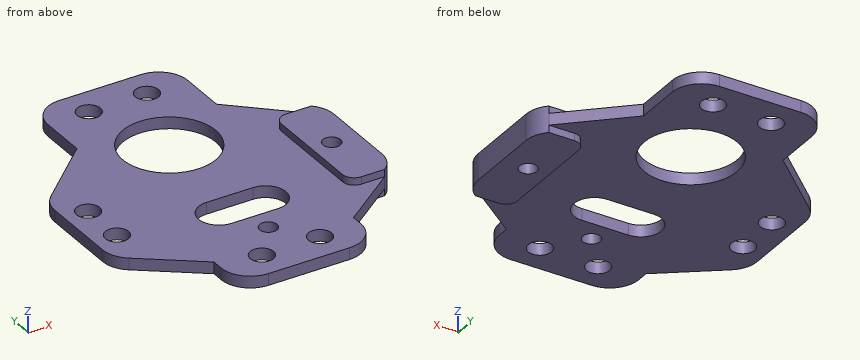
from build123d import *

# Parameters (mm, degrees)
SKETCH_1_R               = 2
SKETCH_1_R_2             = 8
SKETCH_1_R_3             = 1.5
EXTRUDE_1_DEPTH          = 2
EXTRUDE_2_DEPTH          = 3.25
CUT_EXTRUDE_1_DEPTH      = 39.603141342
CUT_EXTRUDE_1_DEPTH_BACK = 39.603141342
SKETCH_3_R               = 1.5
CUT_EXTRUDE_2_DEPTH      = 2
FILLET_1_R               = 2


with BuildPart() as part:
    # 草图1 → 凸台-拉伸1 (new body)
    with BuildSketch(Plane(origin=(0, 0, 0), x_dir=(-1, 0, 0), z_dir=(0, 0, -1))):
        with BuildLine():
            Line((-12.803038101, -22.40151905), (-12.803038101, -24.40151905))
            ThreePointArc((-12.803038101, -24.40151905), (-11.338572007, -27.937052956), (-7.803038101, -29.40151905))
            Line((-7.803038101, -29.40151905), (6.196961899, -29.40151905))
            ThreePointArc((6.196961899, -29.40151905), (9.732495805, -27.937052956), (11.196961899, -24.40151905))
            Line((11.196961899, -24.40151905), (11.196961899, -22.40151905))
            Line((11.196961899, -22.40151905), (21.196961899, -14.90151905))
            ThreePointArc((21.196961899, -14.90151905), (22.669097854, -13.137587028), (23.196961899, -10.90151905))
            Line((23.196961899, -10.90151905), (23.196961899, 2.398972368))
            ThreePointArc((23.196961899, 2.398972368), (22.773702864, 4.412288573), (21.575585042, 6.084743069))
            Line((21.575585042, 6.084743069), (11.196961899, 15.59848095))
            Line((11.196961899, 15.59848095), (11.196961899, 23.59848095))
            ThreePointArc((11.196961899, 23.59848095), (9.732495805, 27.134014855), (6.196961899, 28.59848095))
            Line((6.196961899, 28.59848095), (-7.803038101, 28.59848095))
            ThreePointArc((-7.803038101, 28.59848095), (-11.338572007, 27.134014855), (-12.803038101, 23.59848095))
            Line((-12.803038101, 23.59848095), (-12.803038101, 15.59848095))
            Line((-12.803038101, 15.59848095), (-23.181661243, 6.084743069))
            ThreePointArc((-23.181661243, 6.084743069), (-24.379779065, 4.412288573), (-24.803038101, 2.398972368))
            Line((-24.803038101, 2.398972368), (-24.803038101, -10.90151905))
            ThreePointArc((-24.803038101, -10.90151905), (-24.275174056, -13.137587028), (-22.803038101, -14.90151905))
            Line((-22.803038101, -14.90151905), (-12.803038101, -22.40151905))
        make_face()
        with Locations(Location((19.196961899, -8.40151905, 0), (0, 0, 180))):
            Circle(SKETCH_1_R, mode=Mode.SUBTRACT)
        with Locations(Location((19.196961899, -0.40151905, 0), (0, 0, 180))):
            Circle(SKETCH_1_R, mode=Mode.SUBTRACT)
        with Locations(Location((4.196961899, 23.59848095, 0), (0, 0, 180))):
            Circle(SKETCH_1_R, mode=Mode.SUBTRACT)
        with Locations(Location((-5.803038101, 23.59848095, 0), (0, 0, 180))):
            Circle(SKETCH_1_R, mode=Mode.SUBTRACT)
        with Locations(Location((-0.803038101, 9.34848095, 0), (0, 0, 180))):
            Circle(SKETCH_1_R_2, mode=Mode.SUBTRACT)
        with Locations(Location((-20.803038101, -8.40151905, 0), (0, 0, 180))):
            Circle(SKETCH_1_R, mode=Mode.SUBTRACT)
        with Locations(Location((-20.803038101, -0.40151905, 0), (0, 0, 180))):
            Circle(SKETCH_1_R, mode=Mode.SUBTRACT)
        with Locations(Location((-5.803038101, -24.40151905, 0), (0, 0, 180))):
            Circle(SKETCH_1_R, mode=Mode.SUBTRACT)
        with Locations(Location((4.196961899, -24.40151905, 0), (0, 0, 180))):
            Circle(SKETCH_1_R, mode=Mode.SUBTRACT)
        with Locations(Location((-0.803038101, -18.15151905, 0), (0, 0, 180))):
            Circle(SKETCH_1_R_3, mode=Mode.SUBTRACT)
        with BuildLine():
            Line((3.196961899, -14.40151905), (-4.803038101, -14.40151905))
            ThreePointArc((-4.803038101, -14.40151905), (-8.303038101, -10.90151905), (-4.803038101, -7.40151905))
            Line((-4.803038101, -7.40151905), (3.196961899, -7.40151905))
            ThreePointArc((3.196961899, -7.40151905), (6.696961899, -10.90151905), (3.196961899, -14.40151905))
        make_face(mode=Mode.SUBTRACT)
    extrude(amount=-EXTRUDE_1_DEPTH)

    # 草图2 → 凸台-拉伸2 (add, symmetric)
    with BuildSketch(Plane.XY.offset(2)):
        with BuildLine():
            Line((23.181661243, 6.084743069), (16.803038101, 6.084743069))
            Line((16.803038101, 6.084743069), (16.803038101, -14.90151905))
            Line((16.803038101, -14.90151905), (22.803038101, -14.90151905))
            ThreePointArc((22.803038101, -14.90151905), (24.275174056, -13.137587028), (24.803038101, -10.90151905))
            Line((24.803038101, -10.90151905), (24.803038101, 2.398972368))
            ThreePointArc((24.803038101, 2.398972368), (24.379779065, 4.412288573), (23.181661243, 6.084743069))
        make_face()
    extrude(amount=EXTRUDE_2_DEPTH, both=True)

    # 草图3 → 切除-拉伸1 (cut, two sides: drawn at the far end of the back side and taken through both)
    with BuildSketch(Plane.XY.offset(2).offset(-CUT_EXTRUDE_1_DEPTH_BACK)):
        with Locations((20.303038101, -4.251273341)):
            Circle(SKETCH_3_R)
    extrude(amount=CUT_EXTRUDE_1_DEPTH + CUT_EXTRUDE_1_DEPTH_BACK, mode=Mode.SUBTRACT)

    # 草图4 → 切除-拉伸2 (cut)
    with BuildSketch(Plane.XY.offset(5.25)):
        with BuildLine():
            Line((23.181661243, 6.084743069), (16.803038101, 6.084743069))
            Line((16.803038101, 6.084743069), (16.803038101, -14.90151905))
            Line((16.803038101, -14.90151905), (22.803038101, -14.90151905))
            ThreePointArc((22.803038101, -14.90151905), (24.275174056, -13.137587028), (24.803038101, -10.90151905))
            Line((24.803038101, -10.90151905), (24.803038101, 2.398972368))
            ThreePointArc((24.803038101, 2.398972368), (24.379779065, 4.412288573), (23.181661243, 6.084743069))
        make_face()
    extrude(amount=-CUT_EXTRUDE_2_DEPTH, mode=Mode.SUBTRACT)

    # 圆角1
    fillet_1_edges = [part.edges().sort_by_distance(p)[0] for p in [
        (16.803038101, -14.90151905, 2.625),
        (16.803038101, 6.084743069, 2.625),
        (16.803038101, -14.90151905, -0.625),
        (16.803038101, 6.084743069, -0.625),
    ]]
    fillet(fillet_1_edges, radius=FILLET_1_R)


solid = part.part
Can you work these out from the model? Positions are in its coordinate system, mm. Give positions to 0.01 mm unless a question says otherwise; leave off trailing zeros. Write each loop counter-clockwise with the first axis right and the second up, starting at its lowest first coordinate (ties: lowest second). Pieces come first, ordered by that corner, then holes. Notation, with made-up numbers: M 38.5,-13 L 85.5,-13 A18 ccw 85.5,10 Z; hole C 74,-26.5 d5. An arc over 180 degrees is marked long. Answer in a Markdown table with one row per item. Add a question column.
Item 1: Imagine slicing it at A-A, the plane x = 3. Write out the boundary of the cut face in (y, z).
Item 2: Please list where these lines run through material, in increasing order: L1, parallel to X at y = 23.5, z = 0.4; L2, parallel to Y at x = -18.5, z = 1.5; L3, parallel to Y at x = 8, z = 0.9.
Item 3: Imagine slicing it at B-B, the plane y = 22.5. Write out the boundary of the cut face in (x, z).
Item 4: Imagine slicing it at C-C, the plane x = 18. Write out the boundary of the cut face in (y, z).
Item 5: Imagine slicing it at D-D, the plane x = -12. Write out the boundary of the cut face in (y, z), plus the area to 3 significant figures.
Item 6: For pin 1 Ø4 at (x, y) = (5, 3) entering from -Z; pin 2 Ø1 at (y, z) = (-23.5, 0.5) entering from -X; pin 3 Ø1.4 at (x, z) = (20, 2.5) entering from +Y, each with a flat end and sliding along its axis, tell me the tip position at first contact or that it passes through.
Evaluation:
| question | item | result |
|---|---|---|
| 1 | outline | M -29.4,0 L -14.4,0 L -14.4,2 L -29.4,2 Z; M -7.4,0 L 1.66,0 L 1.66,2 L -7.4,2 Z; M 17.04,0 L 28.6,0 L 28.6,2 L 17.04,2 Z |
| 2 | L1 | x = -11.2 to -6.19, -2.2 to 3.81, 7.8 to 12.8 |
| 2 | L2 | y = -16.92 to -10.28, -6.53 to -2.28, 1.47 to 8.9 |
| 2 | L3 | y = -29.4 to -12.33, -9.48 to 5.86, 12.84 to 28.59 |
| 3 | outline | M -11.2,0 L -5.87,0 L -5.87,2 L -11.2,2 Z; M -2.53,0 L 4.13,0 L 4.13,2 L -2.53,2 Z; M 7.47,0 L 12.8,0 L 12.8,2 L 7.47,2 Z |
| 4 | outline | M -18.5,0 L -14.73,0 L -14.73,-1.25 L 5.92,-1.25 L 5.92,0 L 10.83,0 L 10.83,2 L 5.92,2 L 5.92,3.25 L -14.73,3.25 L -14.73,2 L -18.5,2 Z |
| 5 | outline | M -21.8,0 L 14.86,0 L 14.86,2 L -21.8,2 Z |
| 5 | area | 73.3 mm² |
| 6 | pin 1 | stops at z = 0 |
| 6 | pin 2 | stops at x = -11.2 |
| 6 | pin 3 | stops at y = 9.45 |
